Verification items for the finished model (mm, model axes). Face numbers are marked on the shaded views. Coordinates: 2 decimals unless noted, no trailing zeros. Write each loop counter-clockwise with the first axis right and the second up, starting at its lowest first coordinate (ties: lowest second). Pieces come first, ordered by that corner, then holes.
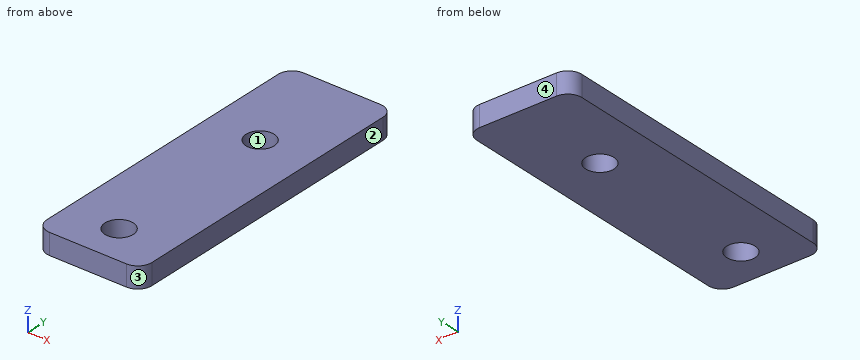
```python
from build123d import *

# Parameters (mm, degrees)
SKETCH_1_W          = 15
SKETCH_1_H          = 45
EXTRUDE_1_DEPTH     = 3
SKETCH_2_R          = 2.025
CUT_EXTRUDE_1_DEPTH = 3
FILLET_1_R          = 2


with BuildPart() as part:
    # 草图1 → 凸台-拉伸1 (new body)
    with BuildSketch(Plane.XY):
        Rectangle(SKETCH_1_W, SKETCH_1_H)
    extrude(amount=EXTRUDE_1_DEPTH)

    # 草图2 → 切除-拉伸1 (cut)
    with BuildSketch(Plane.XY.offset(3)):
        with Locations((0, -17)):
            Circle(SKETCH_2_R)
        with Locations((0, 8)):
            Circle(SKETCH_2_R)
    extrude(amount=-CUT_EXTRUDE_1_DEPTH, mode=Mode.SUBTRACT)

    # 圆角1
    fillet_1_edges = [part.edges().sort_by_distance(p)[0] for p in [
        (7.5, -22.5, 1.5),
        (-7.5, -22.5, 1.5),
        (-7.5, 22.5, 1.5),
        (7.5, 22.5, 1.5),
    ]]
    fillet(fillet_1_edges, radius=FILLET_1_R)


solid = part.part
```
1. Sectioned sample at C-C, the plane y = 8. Record the boundary of the cut face in (x, z) (3 decimals), and give its area (4 significant figures).
2. Draft check along Y on the marked faces 1, 2, 3 and 4. Enter one of: pulls with the +Y half, pulls with the -Y half, needs draft (parallel to the pull), parting line crosses it, or undercut.
3. Sectioned sample at B-B, the plane x = 0. Record the boundary of the cut face in (y, z) (3 decimals).
4. Sectioned sample at A-A, the plane z = 0.6. Record the boundary of the cut face in (x, y) (3 decimals), and give its area (3 significant figures).
5. Material ranges on L1, parallel to Y at x = 0, z = 0.75 (3 decimals); L2, parallel to X at y = 9.5, z = 2.8; L3, parallel to X at y = 7, z = 1, recorded low to high.
Outcome:
1. outline: (-7.5, 0) - (-2.025, 0) - (-2.025, 3) - (-7.5, 3) - close; (2.025, 0) - (7.5, 0) - (7.5, 3) - (2.025, 3) - close
1. area: 32.85 mm2
2. face 1: undercut
2. face 2: needs draft
2. face 3: pulls with the -Y half
2. face 4: pulls with the +Y half
3. outline: (-22.5, 0) - (-19.025, 0) - (-19.025, 3) - (-22.5, 3) - close; (-14.975, 0) - (5.975, 0) - (5.975, 3) - (-14.975, 3) - close; (10.025, 0) - (22.5, 0) - (22.5, 3) - (10.025, 3) - close
4. outline: (-7.5, -20.5) arc R2 ccw to (-5.5, -22.5) - (5.5, -22.5) arc R2 ccw to (7.5, -20.5) - (7.5, 20.5) arc R2 ccw to (5.5, 22.5) - (-5.5, 22.5) arc R2 ccw to (-7.5, 20.5) - close; hole circle Ø4.05 at (0, -17); hole circle Ø4.05 at (0, 8)
4. area: 646 mm2
5. L1: y = -22.5 to -19.025, -14.975 to 5.975, 10.025 to 22.5
5. L2: x = -7.5 to -1.36, 1.36 to 7.5
5. L3: x = -7.5 to -1.76, 1.76 to 7.5
